Can you work these out from the model? Positions are in its coordinate system, mm. A direction names the side the tool comes from. Round coordinates to 2 decimals unless told otherwise and drop trailing zeros. Write each loop counter-clockwise with the first axis right and the second up, starting at its lowest first coordinate (ties: lowest second). Pieces come first, ordered by that corner, then holes. Notation, with made-up numbers: (73.25, 20.25) - (119.25, 20.25) arc R8 cw to (119.25, 28.25) - close; hole circle Ø1 at (43.5, -19). An arc over 180 degrees is marked (long way). One line per item, written item: value. Start each with the question number.
(1) Thinking about a two-plate mould opening in X: for faces 1 (the face through (-26.495, 57.525, 1.479)), 2 (the face through (51.5, 44.807, 1.479)), 3 (the face through (26.9, 57.46, 1.48)), 4 (the face through (-1, -44, 0)), which applies, +X half, -X half, draft (parallel to the pull), parting line (faces both ways), or undercut?
(2) If I drill on L1, parallel to X at y = -25.5, z = 1; L2, parallel to X at y = 2, z = 1.7; L3, parallel to X at y = -172, z = 2.6, over which ranges is the centre line in solid material (lowest first)? Write a range as from..to.
(3) I'm going to push flat-ended pins straight in: pin 1 Ø0.9 at (x, z) = (-23, 1.5) entering from +Y; pin 2 Ø0.9 at (y, z) = (-190.5, 1) entering from -X; pin 3 Ø1.5 at (x, z) = (30, 2.5) entering from -Y. Where does each tip first touch, or does it pass through?
(4) On a 3-axis mill with a long thin cutter (end or side, diameter ignored), from which of +Z, -Z, +X, -X, +Y, -Y can I reach the whole of each face in a straight line? I mean faces 5 (the face through (-1, -44, 3)), 6 (the face through (-19.587, -30.692, 1.479)). Say none if no direction works.
(5) I want a section at D-D on y = -168. List the corners of the cut face in (x, z) for me, plus the area to 3 significant figures.
(6) I want a section at B-B on y = 9. List the corners of the cut face in (x, z) for me, plus the area to 3 significant figures.
(7) I want a section at C-C on z = 0.6. Give the number of separate pieces and of enclosed holes in the cut face, plus the area to 3 significant figures.
(8) I want a section at A-A on x = 50. List the corners of the cut face in (y, z) for me, plus the area to 3 significant figures.
Autodesk Inventor part; units mm, degrees
ref_plane "YZ Plane" through (0, 0, 0) normal (1, 0, 0) x (0, 1, 0)
ref_plane "XZ Plane" through (0, 0, 0) normal (0, 1, 0) x (-1, 0, 0)
ref_plane "XY Plane" through (0, 0, 0) normal (0, 0, 1) x (1, 0, 0)
sketch "Sketch1" plane through (0, 0, 0) normal (0, 0, 1) x (1, 0, 0)
  arc A0 (-20.3204, 17.9615) -> (-32.1264, 16.3566) centre (-26.2234, 17.159) ccw
  line L0 (-20.3204, 17.9615) -> (-14.6157, -24.0052)
  arc A1 (-26.4217, -25.6101) -> (-14.6157, -24.0052) centre (-20.5187, -24.8077) ccw
  line L1 (-26.4217, -25.6101) -> (-32.1264, 16.3566)
  arc A2 (-17.4681, 46.3619) -> (-13.8821, 37.9739) centre (-13.8821, 42.9344) ccw
  arc A3 (17.4681, 46.3619) -> (-17.4681, 46.3619) centre (0, 29.6659) ccw
  arc A4 (13.8821, 37.9739) -> (17.4681, 46.3619) centre (13.8821, 42.9344) ccw
  line L2 (13.8821, 37.9739) -> (-13.8821, 37.9739)
  arc A5 (32.1264, 16.3566) -> (20.3204, 17.9615) centre (26.2234, 17.159) ccw
  line L3 (32.1264, 16.3566) -> (26.4217, -25.6101)
  arc A6 (14.6157, -24.0052) -> (26.4217, -25.6101) centre (20.5187, -24.8077) ccw
  line L4 (14.6157, -24.0052) -> (20.3204, 17.9615)
  circle A7 centre (-28.3016, 42.9344) radius 4
  circle A8 centre (-20.018, -41.0528) radius 4
  circle A9 centre (20.018, -41.0528) radius 4
  circle A10 centre (28.3016, 42.9344) radius 4
  circle A11 centre (-50, 41.9238) radius 3.25
  circle A12 centre (50, 41.9238) radius 3.25
  circle A13 centre (20.018, -66.0762) radius 3.25
  circle A14 centre (-20.018, -66.0762) radius 3.25
  line L5 (64.7409, 50.3067) -> (64.7409, 34.44)
  arc A15 (64.7409, 50.3067) -> (58.7409, 56.3067) centre (58.7409, 50.3067) ccw
  line L6 (41.2562, 56.3067) -> (58.7409, 56.3067)
  arc A16 (12.5221, 61.0169) -> (41.2562, 56.3067) centre (41.2562, 146.3067) ccw
  arc A17 (12.5221, 61.0169) -> (-12.5221, 61.0169) centre (0, 23.8483) ccw
  arc A18 (-41.2562, 56.3067) -> (-12.5221, 61.0169) centre (-41.2562, 146.3067) ccw
  line L7 (-41.2562, 56.3067) -> (-58.7409, 56.3067)
  arc A19 (-58.7409, 56.3067) -> (-64.7409, 50.3067) centre (-58.7409, 50.3067) ccw
  line L8 (-64.7409, 50.3067) -> (-64.7409, 21.44)
  line L9 (-64.7409, 21.44) -> (-64.7409, -66.0762)
  line L10 (22, -123.1517) -> (25, -123.1517)
  line L11 (22, -153.1517) -> (25, -153.1517)
  line L12 (22, -183.1517) -> (25, -183.1517)
  line L13 (22, -213.1517) -> (25, -213.1517)
  line L14 (22, -183.1517) -> (22, -213.1517)
  line L15 (22, -123.1517) -> (22, -153.1517)
  line L16 (25, -153.1517) -> (25, -183.1517)
  line L17 (64.7409, -66.0762) -> (-64.7409, -66.0762) construction
  line L18 (64.7409, 34.44) -> (64.7409, -66.0762)
  line L19 (64.7409, -66.0762) -> (25, -123.1517)
  line L20 (25, -213.1517) -> (25, -216.1517)
  line L21 (25, -216.1517) -> (0, -216.1517)
  line L22 (0, -216.1517) -> (0, -66.0762)
  line L23 (-22, -123.1517) -> (-25, -123.1517)
  line L24 (-22, -153.1517) -> (-25, -153.1517)
  line L25 (-22, -183.1517) -> (-25, -183.1517)
  line L26 (-22, -213.1517) -> (-25, -213.1517)
  line L27 (-22, -183.1517) -> (-22, -213.1517)
  line L28 (-22, -123.1517) -> (-22, -153.1517)
  line L29 (-25, -153.1517) -> (-25, -183.1517)
  line L30 (-64.7409, -66.0762) -> (-25, -123.1517)
  line L31 (-25, -213.1517) -> (-25, -216.1517)
  line L32 (-25, -216.1517) -> (0, -216.1517)
  point P0 (20.018, -66.0762)
  point P1 (-64.7409, -22.3181)
  point P2 (27.0258, 23.062)
  point P3 (64.7409, 42.3734)
  dimension "d5" = 30
  dimension "d6" = 30
  dimension "d7" = 30
  dimension "d10" = 3
  dimension "d11" = 3
  dimension "d12" = 240
  dimension "d13" = 50
extrude "Extrusion1" add sketch "Sketch1" along normal blind 3 contours A3 A4 L2 A2 | L5 L18 L19 L10 L15 L11 L16 L12 L14 L13 L20 L21 L32 L31 L26 L27 L25 L29 L24 L28 L23 L30 L9 L8 A19 L7 A18 A17 A16 L6 A15
sketch "Sketch2" plane through (0, 0, 0) normal (0, 0, -1) x (-1, 0, 0)
  line L0 (-25, -216.1517) -> (25, -216.1517)
  line L1 (-10, -216.1517) -> (10, -216.1517)
  line L2 (10, -216.1517) -> (10, -213.1517)
  line L3 (10, -213.1517) -> (-10, -213.1517)
  line L4 (-10, -213.1517) -> (-10, -216.1517)
  line L5 (0, -213.1517) -> (0, -190.7997)
  point P0 (0, 0)
  dimension "d16" = 20
  dimension "d17" = 3
extrude "Extrusion2" cut sketch "Sketch2" against normal blind 6
properties part number "Arm - stand plate"
Established:
1. face 1: -X half
1. face 2: undercut
1. face 3: +X half
1. face 4: draft
2. L1: -64.74..-26.44, -14.6..14.6, 26.44..64.74
2. L2: -64.74..-30.17, -18.15..18.15, 30.17..64.74
2. L3: -25..25
3. pin 1: y = 58.27
3. pin 2: x = -22
3. pin 3: y = -117.05
4. face 5: +Z, +X, -X, +Y, -Y
4. face 6: +Z, -Z
5. outline: (-25, 0) - (25, 0) - (25, 3) - (-25, 3) - close
5. area: 150 mm2
6. outline: (-64.74, 0) - (-31.13, 0) - (-31.13, 3) - (-64.74, 3) - close; (-19.1, 0) - (19.1, 0) - (19.1, 3) - (-19.1, 3) - close; (31.13, 0) - (64.74, 0) - (64.74, 3) - (31.13, 3) - close
6. area: 316 mm2
7. separate pieces: 1
7. enclosed holes: 10
7. area: 23,900 mm2
8. outline: (-87.25, 0) - (38.67, 0) - (38.67, 3) - (-87.25, 3) - close; (45.17, 0) - (56.31, 0) - (56.31, 3) - (45.17, 3) - close
8. area: 411 mm2
